```python
from build123d import *

# Parameters (mm, degrees)
EXTRUDE_START            = 27
SKETCH_3_R               = 8
EXTRUDE_1_DEPTH          = 27
SKETCH_4_W               = 21.869380784
SKETCH_4_H               = 6.809627549
CUT_EXTRUDE_1_DEPTH      = 23
SKETCH_5_R               = 3.5
CUT_EXTRUDE_2_DEPTH      = 70
PATTERN_CIRCULAR_1_COUNT = 6
HOLE_WIZARD_M41_D        = 4.5
HOLE_WIZARD_M41_DEPTH    = 14
HOLE_WIZARD_M41_TIP      = 1.351936393
SKETCH_14_R              = 9.95061624
SKETCH_14_R_2            = 8
CUT_EXTRUDE_5_DEPTH      = 10


with BuildPart() as part:
    # Эскиз2 → Повернуть1 (revolve)
    with BuildSketch(Plane.XY):
        Polygon((-10, -1.978246769), (-56.333333333, -1.978246769), (-63, -16.978246769), (-63, -53.978246769), (-69, -53.978246769), (-69, -58.978246769), (-34.298944769, -58.978246769), (-25.298944769, -62.978246769), (0, -62.978246769), (0, -2.978246769), (-8, -2.978246769), (-8, -13.730591033), (-10, -13.730591033), align=None)
    revolve(axis=Axis((0, -2.978246769, 0), (0, -1, 0)))

    # Эскиз3 → Бобышка-Вытянуть1 (add)
    with BuildSketch(Plane.XZ.offset(62.978246769).offset(EXTRUDE_START)):
        with Locations(Location((0, 0, 0), (0, 0, 180))):
            Circle(SKETCH_3_R)
    extrude(amount=-EXTRUDE_1_DEPTH)

    # Эскиз4 → Вырез-Вытянуть1 (cut)
    with BuildSketch(Plane.XZ.offset(89.978246769)):
        with Locations((-0.065477188, 8.404813774)):
            Rectangle(SKETCH_4_W, SKETCH_4_H)
    extrude(amount=-CUT_EXTRUDE_1_DEPTH, mode=Mode.SUBTRACT)

    # Эскиз5 → Вырез-Вытянуть2 (cut)
    with BuildSketch(Plane.XZ.offset(89.978246769)):
        with Locations(Location((0, 0, 0), (0, 0, 270))):
            Circle(SKETCH_5_R)
    extrude(amount=-CUT_EXTRUDE_2_DEPTH, mode=Mode.SUBTRACT)

    # Эскиз7 → Зенковка для винта с полупотайной головкой M51 (revolve, cut)
    with BuildSketch(Plane(origin=(-1.157683247, -58.978246769, -60), x_dir=(0, 0, -1), z_dir=(1, 0, 0))):
        Polygon((0, 0), (0, 15.652366702), (2.75, 14), (2.75, 2.45), (5.2, 0), align=None)
    hole_wizard_m51 = revolve(axis=Axis((-1.157683247, -65.328246769, -60), (0, 1, 0)), mode=Mode.SUBTRACT)

    # Круговой массив1: Зенковка для винта с полупотайной головкой M51 ×6 about axis
    pattern_circular_1_axis = Axis((0, 0, 0), (0, 1, 0))
    for i in range(1, PATTERN_CIRCULAR_1_COUNT):
        add(hole_wizard_m51.rotate(pattern_circular_1_axis, i * 360 / PATTERN_CIRCULAR_1_COUNT), mode=Mode.SUBTRACT)

    # Отверстие с зазором M41
    with Locations(Plane(origin=(0, -2.978246769, 0), x_dir=(1, 0, 0), z_dir=(0, 1, 0))):
        with Locations((0, 0)):
            Hole(HOLE_WIZARD_M41_D / 2, depth=HOLE_WIZARD_M41_DEPTH)
            with Locations((0, 0, -(HOLE_WIZARD_M41_DEPTH + HOLE_WIZARD_M41_TIP / 2))):  # 118° drill point
                Cone(0, HOLE_WIZARD_M41_D / 2, HOLE_WIZARD_M41_TIP, mode=Mode.SUBTRACT)

    # Эскиз14 → Вырез-Вытянуть5 (cut)
    with BuildSketch(Plane.XZ.offset(62.978246769)):
        Circle(SKETCH_14_R)
        with Locations(Location((0, 0, 0), (0, 0, 180))):
            Circle(SKETCH_14_R_2, mode=Mode.SUBTRACT)
    extrude(amount=-CUT_EXTRUDE_5_DEPTH, mode=Mode.SUBTRACT)


solid = part.part
```
Input: part model. Units: mm. Frame: model coordinates. A direction names the side the tool comes from. Round coordinates to 2 decimals unless told otherwise and drop trailing zeros. Loops run counter-clockwise (first coordinate to the right, second up) from the corner with the lowest first, then second, coordinate; pieces in that order, holes last. Notation, with made-up numbers: (19.25, 5.25) - (37.25, 5.25) arc R18 ccw to (37.25, 34.25) - close; hole circle Ø1 at (68, 47). An arc over 180 degrees is marked (long way). One line per item, written item: value. Start each with the question number.
(1) Section B-B, the plane y = -83. Return loops of the section in (x, z) (3 decimals).
(2) Draft query along X for faces 5 (the flat face through (-1, -1.978, 12)), 6 (the cylindrical face through (-65.814, -56.513, -20.726)), 7 (the conical face through (-52.72, -43.61, -28.56)). Return one class per face: +X half, -X half, draft (parallel to the pull), parting line (faces both ways), or undercut.
(3) Section A-A, the plane y = -32. Return loops of the section in (x, z), plus the area to 3 significant figures.
(4) Ray query, line 1 (Y direction, x = 35, z = 57.5); line 2 (Y direction, x = -23, z = -44); line 3 (Z direction, x = 37.5, y = -14). Return the intervals inside material, ascending. Write a range as [from, to].
(5) Access query for faces 1 (the cylindrical face through (1.73, -8.43, 7.81)), 2 (the flat face through (-11, -62.978, 0)), 3 (the flat face through (0, -79, 5)), 4 (the flat face through (0, -89.978, -4)). Directions: +Z, -Z, +X, -X, +Y, -Y. A direction counts if a zero-diameter tool reaches every point of the face in a straight line with its end or side. Return the directions, or none.
(6) Contact query for flat-ended pins moving along their axis: P1, Ø16, axis at x = 0, z = 0, coming from the +Y side; P2, Ø3.5, axis at x = -1.16, z = -60, coming from the -Y side; P3, Ø5, axis at x = -35.5, y = -12.5, coming from the +Z side. Output: stop coordinate, or through.
Results below:
1. outline: (-6.245, 5) arc R8 ccw (long way) to (6.245, 5) - close; hole circle Ø7 at (0, 0)
2. face 5: draft
2. face 6: parting line
2. face 7: undercut
3. outline: circle Ø126 at (0, 0); hole circle Ø7 at (0, 0)
3. area: 12,400 mm^2
4. line 1: [-58.98, -53.98]
4. line 2: [-58.98, -1.98]
4. line 3: [-48.97, 48.97]
5. face 1: +Y
5. face 2: -Y
5. face 3: +Z, +X, -X, -Y
5. face 4: +Z, -Z, +X, -X, -Y
6. P1: y = -2.98
6. P2: y = -44.38
6. P3: z = 51.79
